from build123d import *

# Parameters (mm, degrees)
SKETCH1_R           = 10.16
SKETCH1_R_2         = 2.54
BOSS_EXTRUDE1_DEPTH = 3.175


with BuildPart() as part:
    # Sketch1 → Boss-Extrude1 (new body)
    with BuildSketch(Plane(origin=(0, 0, 0), x_dir=(1, 0, 0), z_dir=(0, 1, 0))):
        with BuildLine():
            Line((-28.4999938, 15.7999938), (-28.4999938, 9.525))
            Line((-28.4999938, 9.525), (-36.1199938, 9.525))
            ThreePointArc((-36.1199938, 9.525), (-39.712096248, 8.037102448), (-41.1999938, 4.445))
            Line((-41.1999938, 4.445), (-41.1999938, -4.445))
            ThreePointArc((-41.1999938, -4.445), (-39.712096248, -8.037102448), (-36.1199938, -9.525))
            Line((-36.1199938, -9.525), (-28.4999938, -9.525))
            Line((-28.4999938, -9.525), (-28.4999938, -15.7999938))
            Line((-28.4999938, -15.7999938), (-15.7999938, -15.7999938))
            Line((-15.7999938, -15.7999938), (-15.7999938, -28.4999938))
            Line((-15.7999938, -28.4999938), (15.7999938, -28.4999938))
            Line((15.7999938, -28.4999938), (15.7999938, -15.7999938))
            Line((15.7999938, -15.7999938), (28.4999938, -15.7999938))
            Line((28.4999938, -15.7999938), (28.4999938, -9.525))
            Line((28.4999938, -9.525), (36.1199938, -9.525))
            ThreePointArc((36.1199938, -9.525), (39.712096248, -8.037102448), (41.1999938, -4.445))
            Line((41.1999938, -4.445), (41.1999938, 4.445))
            ThreePointArc((41.1999938, 4.445), (39.712096248, 8.037102448), (36.1199938, 9.525))
            Line((36.1199938, 9.525), (28.4999938, 9.525))
            Line((28.4999938, 9.525), (28.4999938, 15.7999938))
            Line((28.4999938, 15.7999938), (15.7999938, 15.7999938))
            Line((15.7999938, 15.7999938), (15.7999938, 28.4999938))
            Line((15.7999938, 28.4999938), (-15.7999938, 28.4999938))
            Line((-15.7999938, 28.4999938), (-15.7999938, 15.7999938))
            Line((-15.7999938, 15.7999938), (-28.4999938, 15.7999938))
        make_face()
        Circle(SKETCH1_R, mode=Mode.SUBTRACT)
        with Locations((-34.8499938, 0)):
            Circle(SKETCH1_R_2, mode=Mode.SUBTRACT)
        with Locations((34.8499938, 0)):
            Circle(SKETCH1_R_2, mode=Mode.SUBTRACT)
    extrude(amount=BOSS_EXTRUDE1_DEPTH)


solid = part.part
The model under review builds one solid part; all positions refer to its coordinate system, in mm. A direction names the side the tool comes from. Round coordinates to 2 decimals unless told otherwise and drop trailing zeros. Loops run counter-clockwise (first coordinate to the right, second up) from the corner with the lowest first, then second, coordinate; pieces in that order, holes last. Notation, with made-up numbers: (74.5, -9) -> (126.5, -9) arc R27 cw to (126.5, 13) -> close; hole circle Ø2 at (27.5, 80). An arc over 180 degrees is marked (long way). Return JSON: item names as keys, results as strings.
(1) Add section D-D on z = 7. Write out the cut boundary in (x, y) (3 decimals).
Solved:
{"outline": "(-40.511, 0) -> (-7.364, 0) -> (-7.364, 3.175) -> (-40.511, 3.175) -> close; (7.364, 0) -> (40.511, 0) -> (40.511, 3.175) -> (7.364, 3.175) -> close"}
(2) For pin 1 (1.5 mm diameter, centred on y = 2.5, z = 17.5, fed in from -X); pin 2 (1 mm diameter, centred on x = 22, y = 2, fed in from -Z); pin 3 (1 mm diameter, centred on x = -32.5, y = 2, fed in from +Z) (3 decimals), all flat-tipped, find the tip position at first contact; note any pin that passes through.
Solved:
{"pin 1": "x = -15.8", "pin 2": "z = -15.8", "pin 3": "z = 9.525"}
(3) For faces 1 (the flat face through (22, 2, 15.8)), 2 (the flat face through (-15.8, 2, -22)), 3 (the flat face through (0, 2, 28.5)), 4 (the flat face through (-28.5, 2, 13)), 5 (the flat face through (28.5, 2, -13)), list the 3-axis set-ups (+Z, -Z, +X, -X, +Y, -Y) from which the entire face can be reached by the end or side of a thin tool; tool diameter is ignored.
Solved:
{"face 1": "+Z, +X, +Y, -Y", "face 2": "-Z, -X, +Y, -Y", "face 3": "+Z, +X, -X, +Y, -Y", "face 4": "+Z, -X, +Y, -Y", "face 5": "-Z, +X, +Y, -Y"}
(4) For line 1 (X direction, y = 1.1, z = 0); line 2 (X direction, y = 0.95, z = 2); line 3 (Z direction, x = 0, y = 1), list the stretches that pass through material, from the lowest coordinate up.
Solved:
{"line 1": "-41.2 to -37.39, -32.31 to -10.16, 10.16 to 32.31, 37.39 to 41.2", "line 2": "-41.2 to -36.42, -33.28 to -9.96, 9.96 to 33.28, 36.42 to 41.2", "line 3": "-28.5 to -10.16, 10.16 to 28.5"}
(5) Add section B-B on y = 2.15. Write out the cut boundary in (x, z) (3 decimals).
Solved:
{"outline": "(-41.2, -4.445) arc R5.08 ccw to (-36.12, -9.525) -> (-28.5, -9.525) -> (-28.5, -15.8) -> (-15.8, -15.8) -> (-15.8, -28.5) -> (15.8, -28.5) -> (15.8, -15.8) -> (28.5, -15.8) -> (28.5, -9.525) -> (36.12, -9.525) arc R5.08 ccw to (41.2, -4.445) -> (41.2, 4.445) arc R5.08 ccw to (36.12, 9.525) -> (28.5, 9.525) -> (28.5, 15.8) -> (15.8, 15.8) -> (15.8, 28.5) -> (-15.8, 28.5) -> (-15.8, 15.8) -> (-28.5, 15.8) -> (-28.5, 9.525) -> (-36.12, 9.525) arc R5.08 ccw to (-41.2, 4.445) -> close; hole circle Ø5.08 at (-34.85, 0); hole circle Ø20.32 at (0, 0); hole circle Ø5.08 at (34.85, 0)"}
(6) Add section A-A on x = 0. Write out the cut boundary in (y, z) (3 decimals), plus the area to 3 significant figures.
Solved:
{"outline": "(0, -28.5) -> (3.175, -28.5) -> (3.175, -10.16) -> (0, -10.16) -> close; (0, 10.16) -> (3.175, 10.16) -> (3.175, 28.5) -> (0, 28.5) -> close", "area": "116 mm2"}
(7) The part is to be moulded in two halves that separate along X. For faces 6 (the cylindrical face through (-1.323, 1.565, -10.074)), 7 (the flat face through (15.8, 2, 22)), 8 (the cylindrical face through (-32.427, 1.565, -0.763)), 9 (the flat face through (32, 2, 9.525)), say which applies: released by +X, released by -X, zero draft, split by the parting line, or undercut.
Solved:
{"face 6": "undercut", "face 7": "released by +X", "face 8": "undercut", "face 9": "zero draft"}
(8) Add section C-C on z = -1. Write out the cut boundary in (x, y) (3 decimals).
Solved:
{"outline": "(-41.2, 0) -> (-37.185, 0) -> (-37.185, 3.175) -> (-41.2, 3.175) -> close; (-32.515, 0) -> (-10.111, 0) -> (-10.111, 3.175) -> (-32.515, 3.175) -> close; (10.111, 0) -> (32.515, 0) -> (32.515, 3.175) -> (10.111, 3.175) -> close; (37.185, 0) -> (41.2, 0) -> (41.2, 3.175) -> (37.185, 3.175) -> close"}
